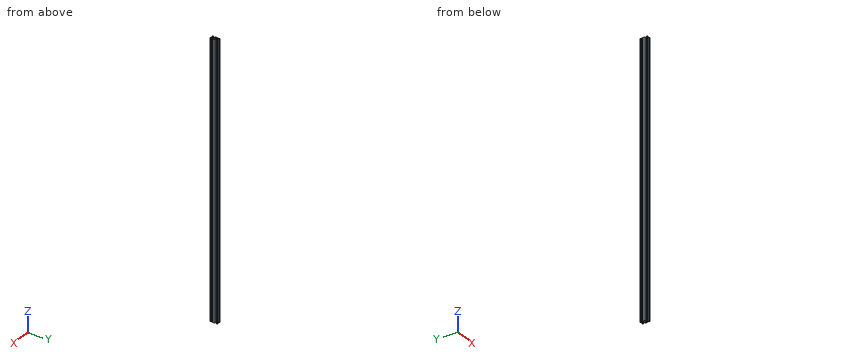
from build123d import *

# Parameters (mm, degrees)
SKETCH2_R           = 2.1
BOSS_EXTRUDE1_DEPTH = 1500


with BuildPart() as part:
    # Sketch2 → Boss-Extrude1 (new body)
    with BuildSketch(Plane.XY):
        with BuildLine():
            Line((-0.1, 3.9), (0, 3.8))
            Line((0, 3.8), (0.1, 3.9))
            Line((0.1, 3.9), (2.840365134, 3.9))
            Line((2.840365134, 3.9), (5.5, 6.558825842))
            Line((5.5, 6.558825842), (5.5, 8.197505675))
            Line((5.5, 8.197505675), (2.89, 8.197505675))
            Line((2.89, 8.197505675), (2.89, 8.307505675))
            Line((2.89, 8.307505675), (4.348614357, 9.766120032))
            ThreePointArc((4.348614357, 9.766120032), (4.604908803, 9.937370505), (4.907228714, 9.997505675))
            Line((4.907228714, 9.997505675), (8.5, 9.997505675))
            ThreePointArc((8.5, 9.997505675), (9.560660172, 9.558165846), (10, 8.497505675))
            Line((10, 8.497505675), (10, 4.904734389))
            ThreePointArc((10, 4.904734389), (9.939864831, 4.602414477), (9.768614357, 4.346120032))
            Line((9.768614357, 4.346120032), (8.31, 2.887505675))
            Line((8.31, 2.887505675), (8.2, 2.887505675))
            Line((8.2, 2.887505675), (8.2, 5.497505675))
            Line((8.2, 5.497505675), (6.56, 5.497505675))
            Line((6.56, 5.497505675), (3.9, 2.83831481))
            Line((3.9, 2.83831481), (3.9, 0.1))
            Line((3.9, 0.1), (3.8, 0))
            Line((3.8, 0), (3.9, -0.1))
            Line((3.9, -0.1), (3.9, -2.84))
            Line((3.9, -2.84), (6.56, -5.5))
            Line((6.56, -5.5), (8.2, -5.5))
            Line((8.2, -5.5), (8.2, -2.89))
            Line((8.2, -2.89), (8.31, -2.89))
            Line((8.31, -2.89), (9.765685425, -4.345685425))
            ThreePointArc((9.765685425, -4.345685425), (9.939103626, -4.605224104), (10, -4.91137085))
            Line((10, -4.91137085), (10, -15.08862915))
            ThreePointArc((10, -15.08862915), (9.939103626, -15.394775896), (9.765685425, -15.654314575))
            Line((9.765685425, -15.654314575), (8.31, -17.11))
            Line((8.31, -17.11), (8.2, -17.11))
            Line((8.2, -17.11), (8.2, -14.5))
            Line((8.2, -14.5), (6.56, -14.5))
            Line((6.56, -14.5), (3.9, -17.16))
            Line((3.9, -17.16), (3.9, -19.9))
            Line((3.9, -19.9), (3.8, -20))
            Line((3.8, -20), (3.9, -20.1))
            Line((3.9, -20.1), (3.9, -22.83831481))
            Line((3.9, -22.83831481), (6.56, -25.497505675))
            Line((6.56, -25.497505675), (8.2, -25.497505675))
            Line((8.2, -25.497505675), (8.2, -22.887505675))
            Line((8.2, -22.887505675), (8.31, -22.887505675))
            Line((8.31, -22.887505675), (9.768614357, -24.346120032))
            ThreePointArc((9.768614357, -24.346120032), (9.939864831, -24.602414477), (10, -24.904734389))
            Line((10, -24.904734389), (10, -28.497505675))
            ThreePointArc((10, -28.497505675), (9.560660172, -29.558165846), (8.5, -29.997505675))
            Line((8.5, -29.997505675), (4.907228714, -29.997505675))
            ThreePointArc((4.907228714, -29.997505675), (4.604908803, -29.937370505), (4.348614357, -29.766120032))
            Line((4.348614357, -29.766120032), (2.89, -28.307505675))
            Line((2.89, -28.307505675), (2.89, -28.197505675))
            Line((2.89, -28.197505675), (5.5, -28.197505675))
            Line((5.5, -28.197505675), (5.5, -26.558825842))
            Line((5.5, -26.558825842), (2.840365134, -23.9))
            Line((2.840365134, -23.9), (0.1, -23.9))
            Line((0.1, -23.9), (0, -23.8))
            Line((0, -23.8), (-0.1, -23.9))
            Line((-0.1, -23.9), (-2.840365134, -23.9))
            Line((-2.840365134, -23.9), (-5.5, -26.558825842))
            Line((-5.5, -26.558825842), (-5.5, -28.197505675))
            Line((-5.5, -28.197505675), (-2.89, -28.197505675))
            Line((-2.89, -28.197505675), (-2.89, -28.307505675))
            Line((-2.89, -28.307505675), (-4.348614357, -29.766120032))
            ThreePointArc((-4.348614357, -29.766120032), (-4.604908803, -29.937370505), (-4.907228714, -29.997505675))
            Line((-4.907228714, -29.997505675), (-8.5, -29.997505675))
            ThreePointArc((-8.5, -29.997505675), (-9.560660172, -29.558165846), (-10, -28.497505675))
            Line((-10, -28.497505675), (-10, -24.904734389))
            ThreePointArc((-10, -24.904734389), (-9.939864831, -24.602414477), (-9.768614357, -24.346120032))
            Line((-9.768614357, -24.346120032), (-8.31, -22.887505675))
            Line((-8.31, -22.887505675), (-8.2, -22.887505675))
            Line((-8.2, -22.887505675), (-8.2, -25.497505675))
            Line((-8.2, -25.497505675), (-6.56, -25.497505675))
            Line((-6.56, -25.497505675), (-3.9, -22.83831481))
            Line((-3.9, -22.83831481), (-3.9, -20.1))
            Line((-3.9, -20.1), (-3.8, -20))
            Line((-3.8, -20), (-3.9, -19.9))
            Line((-3.9, -19.9), (-3.9, -17.16))
            Line((-3.9, -17.16), (-6.56, -14.5))
            Line((-6.56, -14.5), (-8.2, -14.5))
            Line((-8.2, -14.5), (-8.2, -17.11))
            Line((-8.2, -17.11), (-8.31, -17.11))
            Line((-8.31, -17.11), (-9.765685425, -15.654314575))
            ThreePointArc((-9.765685425, -15.654314575), (-9.939103626, -15.394775896), (-10, -15.08862915))
            Line((-10, -15.08862915), (-10, -4.91137085))
            ThreePointArc((-10, -4.91137085), (-9.939103626, -4.605224104), (-9.765685425, -4.345685425))
            Line((-9.765685425, -4.345685425), (-8.31, -2.89))
            Line((-8.31, -2.89), (-8.2, -2.89))
            Line((-8.2, -2.89), (-8.2, -5.5))
            Line((-8.2, -5.5), (-6.56, -5.5))
            Line((-6.56, -5.5), (-3.9, -2.84))
            Line((-3.9, -2.84), (-3.9, -0.1))
            Line((-3.9, -0.1), (-3.8, 0))
            Line((-3.8, 0), (-3.9, 0.1))
            Line((-3.9, 0.1), (-3.9, 2.83831481))
            Line((-3.9, 2.83831481), (-6.56, 5.497505675))
            Line((-6.56, 5.497505675), (-8.2, 5.497505675))
            Line((-8.2, 5.497505675), (-8.2, 2.887505675))
            Line((-8.2, 2.887505675), (-8.31, 2.887505675))
            Line((-8.31, 2.887505675), (-9.768614357, 4.346120032))
            ThreePointArc((-9.768614357, 4.346120032), (-9.939864831, 4.602414477), (-10, 4.904734389))
            Line((-10, 4.904734389), (-10, 8.497505675))
            ThreePointArc((-10, 8.497505675), (-9.560660172, 9.558165846), (-8.5, 9.997505675))
            Line((-8.5, 9.997505675), (-4.907228714, 9.997505675))
            ThreePointArc((-4.907228714, 9.997505675), (-4.604908803, 9.937370505), (-4.348614357, 9.766120032))
            Line((-4.348614357, 9.766120032), (-2.89, 8.307505675))
            Line((-2.89, 8.307505675), (-2.89, 8.197505675))
            Line((-2.89, 8.197505675), (-5.5, 8.197505675))
            Line((-5.5, 8.197505675), (-5.5, 6.558825842))
            Line((-5.5, 6.558825842), (-2.840365134, 3.9))
            Line((-2.840365134, 3.9), (-0.1, 3.9))
        make_face()
        Circle(SKETCH2_R, mode=Mode.SUBTRACT)
        with Locations((0, -20)):
            Circle(SKETCH2_R, mode=Mode.SUBTRACT)
        Polygon((-7.66, 6.567505675), (-6.57, 7.657505675), (-6.57, 8.197505675), (-8.2, 8.197505675), (-8.2, 6.567505675), align=None, mode=Mode.SUBTRACT)
        Polygon((-0.1, -3.9), (0, -3.8), (0.1, -3.9), (2.840365134, -3.9), (6.24, -7.299634866), (8.2, -7.299634866), (8.2, -12.700365134), (6.24, -12.700365134), (2.840365134, -16.1), (0.1, -16.1), (0, -16.2), (-0.1, -16.1), (-2.840365134, -16.1), (-6.24, -12.700365134), (-8.2, -12.700365134), (-8.2, -7.299634866), (-6.24, -7.299634866), (-2.840365134, -3.9), align=None, mode=Mode.SUBTRACT)
        Polygon((8.2, 6.567505675), (7.66, 6.567505675), (6.57, 7.657505675), (6.57, 8.197505675), (8.2, 8.197505675), align=None, mode=Mode.SUBTRACT)
        Polygon((7.66, -26.567505675), (6.57, -27.657505675), (6.57, -28.197505675), (8.2, -28.197505675), (8.2, -26.567505675), align=None, mode=Mode.SUBTRACT)
        Polygon((-8.2, -26.567505675), (-7.66, -26.567505675), (-6.57, -27.657505675), (-6.57, -28.197505675), (-8.2, -28.197505675), align=None, mode=Mode.SUBTRACT)
    extrude(amount=-BOSS_EXTRUDE1_DEPTH)


solid = part.part
Source: CAD feature listing. Evaluate the final solid. Frame: model axes, mm. Round coordinates to 2 decimals unless told otherwise and drop trailing zeros. Use a Markdown table: item, result. Add a question column.
1. First-contact query: pin 1 (4 mm diameter, centred on y = -17.5, z = -428.5, fed in from +X); pin 2 (8 mm diameter, centred on x = -0.5, z = -194.5, fed in from +Y); pin 3 (2 mm diameter, centred on y = -2, z = -1018.5, fed in from +X); pin 4 (4 mm diameter, centred on x = 0, y = 0, fed in from +Z). Flat tips, straight axial feed; report the tip coordinate or a pass-through.
2. Section query A-A (z = -581.5). Give the number of separate pieces and of enclosed holes in the cut face, then the cut area to 3 significant figures.
3. Line query: probe 1 along X at (y, z) = (-27.5, -246); probe 2 along Y at (x, z) = (0, -473.5); probe 3 along Y at (x, z) = (-3, -771). Output: solid intervals per line, ascending.
Derived:
| question | item | result |
|---|---|---|
| 1 | pin 1 | x = 9.89 |
| 1 | pin 2 | y = 9.88 |
| 1 | pin 3 | x = 8.42 |
| 1 | pin 4 | through |
| 2 | separate pieces | 1 |
| 2 | enclosed holes | 7 |
| 2 | area | 291 mm2 |
| 3 | probe 1 | -10 to -8.2, -6.73 to -5.5, 5.5 to 6.73, 8.2 to 10 |
| 3 | probe 2 | -23.8 to -22.1, -17.9 to -16.2, -3.8 to -2.1, 2.1 to 3.8 |
| 3 | probe 3 | -28.42 to -28.2, -24.06 to -15.94, -4.06 to 4.06, 8.2 to 8.42 |
